```python
from build123d import *

# Parameters (mm, degrees)
SKETCH1_R           = 14.25
SKETCH1_R_2         = 2
SKETCH1_R_3         = 1.6
BOSS_EXTRUDE1_DEPTH = 0.75


with BuildPart() as part:
    # Sketch1 → Boss-Extrude1 (new, symmetric)
    with BuildSketch(Plane(origin=(0, 0, 0), x_dir=(1, 0, 0), z_dir=(0, 1, 0))):
        with BuildLine():
            Line((-34.937302436, 52.743938431), (-52.743938431, 34.937302436))
            ThreePointArc((-52.743938431, 34.937302436), (-54.111197998, 32.382898574), (-53.832221535, 29.499055662))
            ThreePointArc((-53.832221535, 29.499055662), (-48, 0), (-53.832221535, -29.499055662))
            ThreePointArc((-53.832221535, -29.499055662), (-54.111197998, -32.382898574), (-52.743938431, -34.937302436))
            Line((-52.743938431, -34.937302436), (-34.937302436, -52.743938431))
            ThreePointArc((-34.937302436, -52.743938431), (-32.382898574, -54.111197998), (-29.499055662, -53.832221535))
            ThreePointArc((-29.499055662, -53.832221535), (0, -48), (29.499055662, -53.832221535))
            ThreePointArc((29.499055662, -53.832221535), (32.382898574, -54.111197998), (34.937302436, -52.743938431))
            Line((34.937302436, -52.743938431), (52.743938431, -34.937302436))
            ThreePointArc((52.743938431, -34.937302436), (54.111197998, -32.382898574), (53.832221535, -29.499055662))
            ThreePointArc((53.832221535, -29.499055662), (48, 0), (53.832221535, 29.499055662))
            ThreePointArc((53.832221535, 29.499055662), (54.111197998, 32.382898574), (52.743938431, 34.937302436))
            Line((52.743938431, 34.937302436), (34.937302436, 52.743938431))
            ThreePointArc((34.937302436, 52.743938431), (32.382898574, 54.111197998), (29.499055662, 53.832221535))
            ThreePointArc((29.499055662, 53.832221535), (0, 48), (-29.499055662, 53.832221535))
            ThreePointArc((-29.499055662, 53.832221535), (-32.382898574, 54.111197998), (-34.937302436, 52.743938431))
        make_face()
        with Locations(Location((0, 0, 0), (0, 0, 90))):
            Circle(SKETCH1_R, mode=Mode.SUBTRACT)
        with Locations(Location((-32.2, 0, 0), (0, 0, 90))):
            Circle(SKETCH1_R_2, mode=Mode.SUBTRACT)
        with Locations(Location((-20.400030637, 31.925871171, 0), (0, 0, 90))):
            Circle(SKETCH1_R_3, mode=Mode.SUBTRACT)
        with Locations(Location((-32.067292527, 48.542880528, 0), (0, 0, 90))):
            Circle(SKETCH1_R_3, mode=Mode.SUBTRACT)
        with Locations(Location((-31.925871171, -20.400030637, 0), (0, 0, 90))):
            Circle(SKETCH1_R_3, mode=Mode.SUBTRACT)
        with Locations(Location((-48.542880528, -32.067292527, 0), (0, 0, 90))):
            Circle(SKETCH1_R_3, mode=Mode.SUBTRACT)
        with Locations(Location((20.400030637, -31.925871171, 0), (0, 0, 90))):
            Circle(SKETCH1_R_3, mode=Mode.SUBTRACT)
        with Locations(Location((32.067292527, -48.542880528, 0), (0, 0, 90))):
            Circle(SKETCH1_R_3, mode=Mode.SUBTRACT)
        with Locations(Location((31.925871171, 20.400030637, 0), (0, 0, 90))):
            Circle(SKETCH1_R_3, mode=Mode.SUBTRACT)
        with Locations(Location((48.542880528, 32.067292527, 0), (0, 0, 90))):
            Circle(SKETCH1_R_3, mode=Mode.SUBTRACT)
        with Locations(Location((32.067292527, 48.542880528, 0), (0, 0, 90))):
            Circle(SKETCH1_R_3, mode=Mode.SUBTRACT)
        with Locations(Location((20.400030637, 31.925871171, 0), (0, 0, 90))):
            Circle(SKETCH1_R_3, mode=Mode.SUBTRACT)
        with Locations(Location((48.542880528, -32.067292527, 0), (0, 0, 90))):
            Circle(SKETCH1_R_3, mode=Mode.SUBTRACT)
        with Locations(Location((31.925871171, -20.400030637, 0), (0, 0, 90))):
            Circle(SKETCH1_R_3, mode=Mode.SUBTRACT)
        with Locations(Location((-32.067292527, -48.542880528, 0), (0, 0, 90))):
            Circle(SKETCH1_R_3, mode=Mode.SUBTRACT)
        with Locations(Location((-20.400030637, -31.925871171, 0), (0, 0, 90))):
            Circle(SKETCH1_R_3, mode=Mode.SUBTRACT)
        with Locations(Location((-48.542880528, 32.067292527, 0), (0, 0, 90))):
            Circle(SKETCH1_R_3, mode=Mode.SUBTRACT)
        with Locations(Location((-31.925871171, 20.400030637, 0), (0, 0, 90))):
            Circle(SKETCH1_R_3, mode=Mode.SUBTRACT)
        with Locations(Location((0, 32.2, 0), (0, 0, 90))):
            Circle(SKETCH1_R_2, mode=Mode.SUBTRACT)
        with Locations(Location((0, -32.2, 0), (0, 0, 90))):
            Circle(SKETCH1_R_2, mode=Mode.SUBTRACT)
        with Locations(Location((32.2, 0, 0), (0, 0, 90))):
            Circle(SKETCH1_R_2, mode=Mode.SUBTRACT)
        with BuildLine():
            Line((9.5, -27.7), (-9.5, -27.7))
            ThreePointArc((-9.5, -27.7), (-14.25, -22.95), (-9.5, -18.2))
            Line((-9.5, -18.2), (9.5, -18.2))
            ThreePointArc((9.5, -18.2), (14.25, -22.95), (9.5, -27.7))
        make_face(mode=Mode.SUBTRACT)
        with BuildLine():
            Line((11.6, -42), (-11.6, -42))
            ThreePointArc((-11.6, -42), (-14.25, -39.35), (-11.6, -36.7))
            Line((-11.6, -36.7), (11.6, -36.7))
            ThreePointArc((11.6, -36.7), (14.25, -39.35), (11.6, -42))
        make_face(mode=Mode.SUBTRACT)
        with BuildLine():
            Line((32.385490578, -25.102290732), (39.951533137, -32.668333291))
            ThreePointArc((39.951533137, -32.668333291), (39.951533137, -39.951533137), (32.668333291, -39.951533137))
            Line((32.668333291, -39.951533137), (25.102290732, -32.385490578))
            ThreePointArc((25.102290732, -32.385490578), (25.102290732, -25.102290732), (32.385490578, -25.102290732))
        make_face(mode=Mode.SUBTRACT)
        with BuildLine():
            Line((-9.5, 27.7), (9.5, 27.7))
            ThreePointArc((9.5, 27.7), (14.25, 22.95), (9.5, 18.2))
            Line((9.5, 18.2), (-9.5, 18.2))
            ThreePointArc((-9.5, 18.2), (-14.25, 22.95), (-9.5, 27.7))
        make_face(mode=Mode.SUBTRACT)
        with BuildLine():
            Line((-11.6, 42), (11.6, 42))
            ThreePointArc((11.6, 42), (14.25, 39.35), (11.6, 36.7))
            Line((11.6, 36.7), (-11.6, 36.7))
            ThreePointArc((-11.6, 36.7), (-14.25, 39.35), (-11.6, 42))
        make_face(mode=Mode.SUBTRACT)
        with BuildLine():
            Line((-32.385490578, 25.102290732), (-39.951533137, 32.668333291))
            ThreePointArc((-39.951533137, 32.668333291), (-39.951533137, 39.951533137), (-32.668333291, 39.951533137))
            Line((-32.668333291, 39.951533137), (-25.102290732, 32.385490578))
            ThreePointArc((-25.102290732, 32.385490578), (-25.102290732, 25.102290732), (-32.385490578, 25.102290732))
        make_face(mode=Mode.SUBTRACT)
        with BuildLine():
            Line((25.102290732, 32.385490578), (32.668333291, 39.951533137))
            ThreePointArc((32.668333291, 39.951533137), (39.951533137, 39.951533137), (39.951533137, 32.668333291))
            Line((39.951533137, 32.668333291), (32.385490578, 25.102290732))
            ThreePointArc((32.385490578, 25.102290732), (25.102290732, 25.102290732), (25.102290732, 32.385490578))
        make_face(mode=Mode.SUBTRACT)
        with BuildLine():
            Line((-25.102290732, -32.385490578), (-32.668333291, -39.951533137))
            ThreePointArc((-32.668333291, -39.951533137), (-39.951533137, -39.951533137), (-39.951533137, -32.668333291))
            Line((-39.951533137, -32.668333291), (-32.385490578, -25.102290732))
            ThreePointArc((-32.385490578, -25.102290732), (-25.102290732, -25.102290732), (-25.102290732, -32.385490578))
        make_face(mode=Mode.SUBTRACT)
        with BuildLine():
            Line((-42, -11.6), (-42, 11.6))
            ThreePointArc((-42, 11.6), (-39.35, 14.25), (-36.7, 11.6))
            Line((-36.7, 11.6), (-36.7, -11.6))
            ThreePointArc((-36.7, -11.6), (-39.35, -14.25), (-42, -11.6))
        make_face(mode=Mode.SUBTRACT)
        with BuildLine():
            Line((-27.7, -9.5), (-27.7, 9.5))
            ThreePointArc((-27.7, 9.5), (-22.95, 14.25), (-18.2, 9.5))
            Line((-18.2, 9.5), (-18.2, -9.5))
            ThreePointArc((-18.2, -9.5), (-22.95, -14.25), (-27.7, -9.5))
        make_face(mode=Mode.SUBTRACT)
        with BuildLine():
            Line((42, 11.6), (42, -11.6))
            ThreePointArc((42, -11.6), (39.35, -14.25), (36.7, -11.6))
            Line((36.7, -11.6), (36.7, 11.6))
            ThreePointArc((36.7, 11.6), (39.35, 14.25), (42, 11.6))
        make_face(mode=Mode.SUBTRACT)
        with BuildLine():
            Line((27.7, 9.5), (27.7, -9.5))
            ThreePointArc((27.7, -9.5), (22.95, -14.25), (18.2, -9.5))
            Line((18.2, -9.5), (18.2, 9.5))
            ThreePointArc((18.2, 9.5), (22.95, 14.25), (27.7, 9.5))
        make_face(mode=Mode.SUBTRACT)
    extrude(amount=BOSS_EXTRUDE1_DEPTH, both=True)


solid = part.part
```
Input: part model. Units: mm. Frame: model coordinates. Give positions to 0.01 mm unless a question says otherwise; leave off trailing zeros. Order: outer loops, then holes, each group sorted by start corner. A loop starts at its lowest first (then second) coordinate and runs counter-clockwise, first axis right, second up. Notation, with made-up numbers: M -23,9.5 L 29,9.5 A16 ccw 29,32.5 Z; hole C 50,17 d4. An arc over 180 degrees is marked long. Return JSON: item names as keys, results as strings.
1) Section query B-B on z = -13. Output: boundary loops of the cut face in (x, y).
Taken from the geometry:
{"outline": "M -49.1,-0.75 L -41.6,-0.75 L -41.6,0.75 L -49.1,0.75 Z; M -37.1,-0.75 L -26.16,-0.75 L -26.16,0.75 L -37.1,0.75 Z; M -19.74,-0.75 L -5.84,-0.75 L -5.84,0.75 L -19.74,0.75 Z; M 5.84,-0.75 L 19.74,-0.75 L 19.74,0.75 L 5.84,0.75 Z; M 26.16,-0.75 L 37.1,-0.75 L 37.1,0.75 L 26.16,0.75 Z; M 41.6,-0.75 L 49.1,-0.75 L 49.1,0.75 L 41.6,0.75 Z"}
2) Line query: L1, parallel to Z at x = -21, y = -0.25; L2, parallel to Z at x = -12.5, y = 0.2; L3, parallel to Z at x = -26, y = -0.35. Output: solid intervals per line, ascending. Write a range as [from, to].
Taken from the geometry:
{"L1": "z = [-50.9, -33.41], [-30.44, -13.83], [13.83, 30.44], [33.41, 50.9]", "L2": "z = [-49.01, -41.84], [-36.86, -26.63], [-19.27, -6.84], [6.84, 19.27], [26.63, 36.86], [41.84, 49.01]", "L3": "z = [-52.49, -33.28], [-24.39, -13.14], [13.14, 24.39], [33.28, 52.49]"}
3) Mould query, pull axis X, two halves, no side actions, for faces 1 (the face through (-40, 0, -39.9)), 2 (the face through (-48, 0, 0)), 3 (the face through (0.766, -0.01, 30.353)). Classes: released by +X, released by -X, zero draft, split by the parting line, or undercut.
Taken from the geometry:
{"face 1": "undercut", "face 2": "released by -X", "face 3": "undercut"}
4) Section query C-C on x = 44. Output: boundary loops of the cut face in (y, z).
Taken from the geometry:
{"outline": "M -0.75,-43.68 L 0.75,-43.68 L 0.75,43.68 L -0.75,43.68 Z"}
5) Section query A-A on x = 0. Count the separate pieces of the cut face and the enclosed holes in it, and give its area (4 significant figures).
Taken from the geometry:
{"separate pieces": "8", "enclosed holes": "0", "area": "44.85 mm2"}
